Part print with two shaded views. Sizes in mm from the minimum x, y, z corner. A direction names the side the tool comes from. Coordinates: 2 decimals unless noted, no trailing zeros. Loops run counter-clockwise (first coordinate to the right, second up) from the corner with the lowest first, then second, coordinate; pieces in that order, holes last. Notation, with made-up numbers: (27, 42.5) -> (43, 42.5) arc R30 cw to (43, 70.5) -> close; hole circle Ø2 at (54, 9). An arc over 180 degrees is marked (long way). Answer as a JSON object with one key per item and string values. Group by question number.
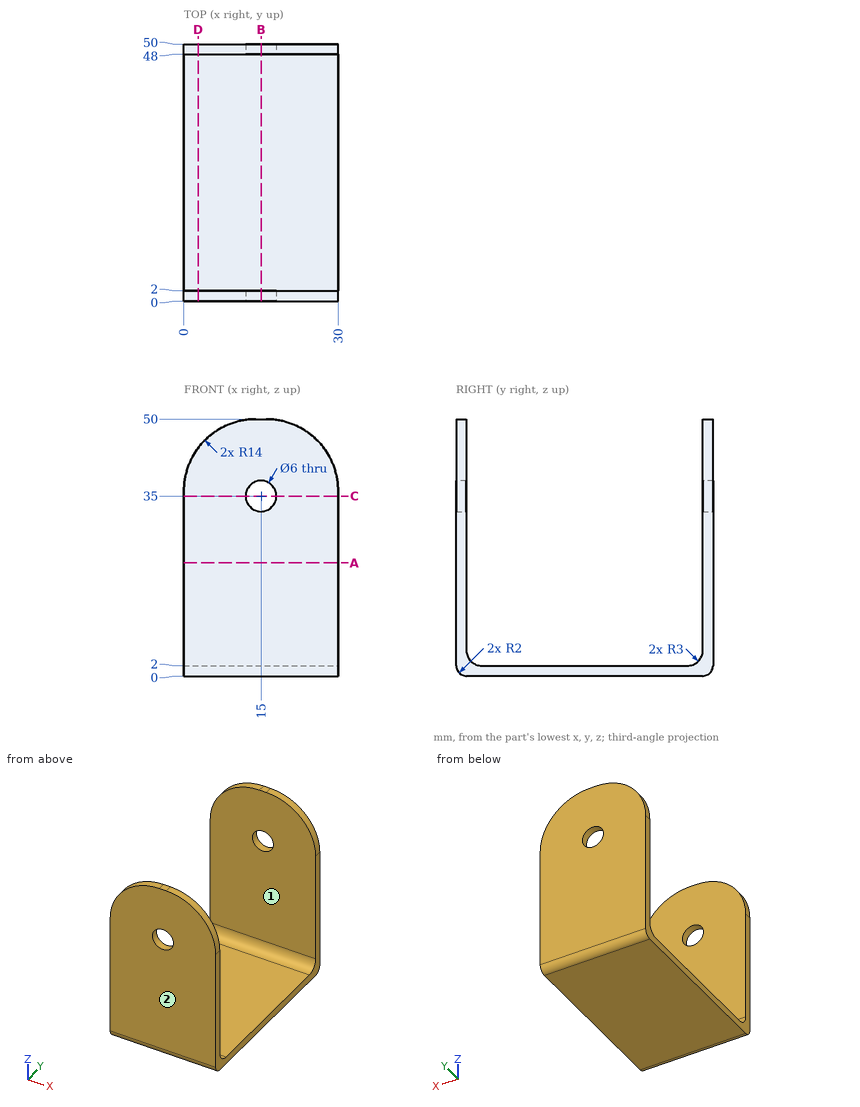
Item 1: Band-saw the part on A-A, the plane z = 22. List the corners of the cut face in (x, y), and give its area (3 significant figures).
Item 2: Band-saw the part on D-D, the plane x = 2.75. List the corners of the cut face in (y, z).
Item 3: Band-saw the part on C-C, the plane z = 35. List the corners of the cut face in (x, y).
Item 4: Drill centre lines: L1, parallel to X at y = 0.9, z = 35; L2, parallel to Y at x = 23, z = 19; L3, parallel to Z at x = 17.5, y = 6.5. Where is each one in solid material? Low to high.
Item 5: Band-saw the part on B-B, the plane x = 15. List the corners of the cut face in (y, z), and give its area (3 significant figures).
Item 6: Flat gauge pin, fed straight in: P1, Ø12, axis at x = 11, y = 20.5, coming from the +Z side. Where does the tip first touch, or does it go through?
Item 7: 3-axis set-ups, long thin cutter, end or side, ignore diameter. For the marked faces 1 and 2: which of +Z, -Z, +X, -X, +Y, -Y reach the whole face in a straight line?
Reply:
{
 "1": {"outline": "(0, 0) -> (30, 0) -> (30, 2) -> (0, 2) -> close; (0, 48) -> (30, 48) -> (30, 50) -> (0, 50) -> close", "area": "120 mm²"},
 "2": {"outline": "(0, 2) arc R2 ccw to (2, 0) -> (48, 0) arc R2 ccw to (50, 2) -> (50, 44.33) -> (48, 44.33) -> (48, 5) arc R3 cw to (45, 2) -> (5, 2) arc R3 cw to (2, 5) -> (2, 44.33) -> (0, 44.33) -> close"},
 "3": {"outline": "(0, 0) -> (12, 0) -> (12, 2) -> (0, 2) -> close; (0, 48) -> (12, 48) -> (12, 50) -> (0, 50) -> close; (18, 0) -> (30, 0) -> (30, 2) -> (18, 2) -> close; (18, 48) -> (30, 48) -> (30, 50) -> (18, 50) -> close"},
 "4": {"L1": "0 to 12, 18 to 30", "L2": "0 to 2, 48 to 50", "L3": "0 to 2"},
 "5": {"outline": "(0, 2) arc R2 ccw to (2, 0) -> (48, 0) arc R2 ccw to (50, 2) -> (50, 32) -> (48, 32) -> (48, 5) arc R3 cw to (45, 2) -> (5, 2) arc R3 cw to (2, 5) -> (2, 32) -> (0, 32) -> close; (0, 38) -> (2, 38) -> (2, 50) -> (0, 50) -> close; (48, 38) -> (50, 38) -> (50, 50) -> (48, 50) -> close", "area": "270 mm²"},
 "6": {"P1": "z = 2"},
 "7": {"face 1": "+Z, +X, -X", "face 2": "+Z, -Z, +X, -X, -Y"}
}
